Verification items for the finished model (mm, model axes). A direction names the side the tool comes from. Give positions to 0.01 mm unless a question says otherwise; leave off trailing zeros. Write each loop counter-clockwise with the first axis right and the second up, starting at its lowest first coordinate (ties: lowest second). Pieces come first, ordered by that corner, then holes. Notation, with made-up numbers: M 43,-18.75 L 60,-18.75 A13 cw 60,-11.75 Z; hole C 27,-1 d1. An arc over 180 degrees is marked long. Write item = value, one per line.
from build123d import *

# Parameters (mm, degrees)
SKETCH1_R             = 34.6075
SKETCH1_R_2           = 26.67
BOSS_EXTRUDE1_DEPTH   = 226.06
BOSS_EXTRUDE2_START   = -12.7
BOSS_EXTRUDE2_DEPTH   = 3.175
BOSS_EXTRUDE2_START_2 = 9.525
BOSS_EXTRUDE2_2_DEPTH = 3.175
BOSS_EXTRUDE2_START_3 = -9.525
BOSS_EXTRUDE2_3_DEPTH = 19.05
SKETCH3_R             = 50.8
SKETCH3_R_2           = 38.1
BOSS_EXTRUDE3_DEPTH   = 38.1


# Read off the part's stored shape, not the designer's step: Boss-Extrude2
with BuildPart() as part:
    # Sketch1 → Boss-Extrude1 (new, symmetric)
    with BuildSketch(Plane.XY):
        with Locations(Location((0, 0, 0), (0, 0, 180))):
            Circle(SKETCH1_R)
        with Locations(Location((0, 0, 0), (0, 0, 180))):
            Circle(SKETCH1_R_2, mode=Mode.SUBTRACT)
    extrude(amount=BOSS_EXTRUDE1_DEPTH, both=True)

    # Boss-Extrude2 outline → Boss-Extrude2 (add)
    with BuildSketch(Plane.XY.offset(BOSS_EXTRUDE2_START)):
        with BuildLine():
            Line((861.705723904, 25.4), (23.505723904, 25.4))
            ThreePointArc((23.505723904, 25.4), (34.6075, 0), (23.505723904, -25.4))
            Line((23.505723904, -25.4), (861.705723904, -25.4))
            ThreePointArc((861.705723904, -25.4), (872.8075, 0), (861.705723904, 25.4))
        make_face()
    extrude(amount=BOSS_EXTRUDE2_DEPTH)

    # Boss-Extrude2 2 outline → Boss-Extrude2 2 (add)
    with BuildSketch(Plane.XY.offset(BOSS_EXTRUDE2_START_2)):
        with BuildLine():
            Line((861.705723904, 25.4), (23.505723904, 25.4))
            ThreePointArc((23.505723904, 25.4), (34.6075, 0), (23.505723904, -25.4))
            Line((23.505723904, -25.4), (861.705723904, -25.4))
            ThreePointArc((861.705723904, -25.4), (872.8075, 0), (861.705723904, 25.4))
        make_face()
    extrude(amount=BOSS_EXTRUDE2_2_DEPTH)

    # Boss-Extrude2 3 outline → Boss-Extrude2 3 (add)
    with BuildSketch(Plane.XY.offset(BOSS_EXTRUDE2_START_3)):
        with BuildLine():
            ThreePointArc((864.727880263, 22.225), (863.267120751, 23.86039634), (861.705723904, 25.4))
            Line((861.705723904, 25.4), (23.505723904, 25.4))
            ThreePointArc((23.505723904, 25.4), (25.067120751, 23.86039634), (26.527880263, 22.225))
            Line((26.527880263, 22.225), (864.727880263, 22.225))
        make_face()
        with BuildLine():
            ThreePointArc((861.705723904, -25.4), (863.267120751, -23.86039634), (864.727880263, -22.225))
            Line((864.727880263, -22.225), (26.527880263, -22.225))
            ThreePointArc((26.527880263, -22.225), (25.067120751, -23.86039634), (23.505723904, -25.4))
            Line((23.505723904, -25.4), (861.705723904, -25.4))
        make_face()
    extrude(amount=BOSS_EXTRUDE2_3_DEPTH)

    # Sketch3 → Boss-Extrude3 (add, symmetric)
    with BuildSketch(Plane(origin=(0, 0, 0), x_dir=(1, 0, 0), z_dir=(0, 1, 0))):
        with Locations(Location((914.4, 0, 0), (0, 0, 270))):
            Circle(SKETCH3_R)
        with Locations(Location((914.4, 0, 0), (0, 0, 90))):
            Circle(SKETCH3_R_2, mode=Mode.SUBTRACT)
    extrude(amount=BOSS_EXTRUDE3_DEPTH, both=True)


solid = part.part
1) Depth check by flat-ended pin: P1, Ø15, axis at x = 590.5, z = 4, coming from the +Y side; P2, Ø8, axis at x = 308.5, y = -4, coming from the -Z side; P3, Ø3, axis at y = 13.5, z = 87.5, coming from the +X side. Enter the tip coordinate at first touch or a pass-through.
From the geometry:
P1 = 25.4
P2 = -12.7
P3 = 32.46
2) Tool access check on faces 1 (the cylindrical face through (3.472, -26.443, -3.165)), 2 (the flat face through (448, 25.4, 0)), 3 (the flat face through (440, 22.225, 0)). Record the directions out of +Z, -Z, +X, -X, +Y, -Y that give a thin tool (end or side, any length) a straight path to the whole face; none if there is none.
From the geometry:
face_1 = +Z, -Z
face_2 = +Z, -Z, +Y
face_3 = none
3) Cross-section at A-A on y = 0. Record the boundary of the cut face in (x, z) (1 decimal).
From the geometry:
outline = M -34.6,-226.1 L -26.7,-226.1 L -26.7,226.1 L -34.6,226.1 Z; M 26.7,-226.1 L 34.6,-226.1 L 34.6,-12.7 L 865.2,-12.7 A50.8 ccw long 865.2,12.7 L 34.6,12.7 L 34.6,226.1 L 26.7,226.1 Z; hole M 34.6,-9.5 L 864.5,-9.5 A50.8 cw 864.5,9.5 L 34.6,9.5 Z; hole C 914.4,0 d76.2
4) Draft check along X on faces 4 (the flat face through (-18, 20, 226.06)), 5 (the flat face through (437, -25.4, 0)). Enter one of: +X half, -X half, draft (parallel to the pull), parting line (faces both ways), or undercut.
From the geometry:
face_4 = draft
face_5 = undercut
5) Cross-section at C-C on z = 0. Record the boundary of the cut face in (x, y) (1 decimal).
From the geometry:
outline = M 23.5,-25.4 L 861.7,-25.4 A34.6 ccw 863.6,-23.5 L 863.6,-38.1 L 876.3,-38.1 L 876.3,38.1 L 863.6,38.1 L 863.6,23.5 A34.6 ccw 861.7,25.4 L 23.5,25.4 A34.6 ccw long Z; M 952.5,-38.1 L 965.2,-38.1 L 965.2,38.1 L 952.5,38.1 Z; hole C 0,0 d53.3; hole M 26.5,-22.2 L 863.6,-22.2 L 863.6,22.2 L 26.5,22.2 A34.6 cw Z
6) Cross-section at B-B on x = 914.4. Record the boundary of the cut face in (y, z).
From the geometry:
outline = M -38.1,-50.8 L 38.1,-50.8 L 38.1,-38.1 L -38.1,-38.1 Z; M -38.1,38.1 L 38.1,38.1 L 38.1,50.8 L -38.1,50.8 Z
7) Material ranges on probe 1 along Z at (x, y) = (914, 7); probe 2 along X at (y, z) = (3, -74.5); probe 3 along Z at (x, y) = (541, -6) (3 decimals), recorded low to high. Write a range as from..to.
From the geometry:
probe_1 = -50.8..-38.1, 38.1..50.8
probe_2 = -34.48..-26.5, 26.5..34.48
probe_3 = -12.7..-9.525, 9.525..12.7
8) Cross-section at D-D on x = 398.5. Record the boundary of the cut face in (y, z) (3 decimals).
From the geometry:
outline = M -25.4,-12.7 L 25.4,-12.7 L 25.4,12.7 L -25.4,12.7 Z; hole M -22.225,-9.525 L 22.225,-9.525 L 22.225,9.525 L -22.225,9.525 Z
